Source: three-view drawing plus pictorial views. Frame: mm from the lowest corner of the part. A direction names the side the tool comes from. Give positions to 0.01 mm unless a question says otherwise; leave off trailing zeros. Loops run counter-clockwise (first coordinate to the right, second up) from the corner with the lowest first, then second, coordinate; pieces in that order, holes last.
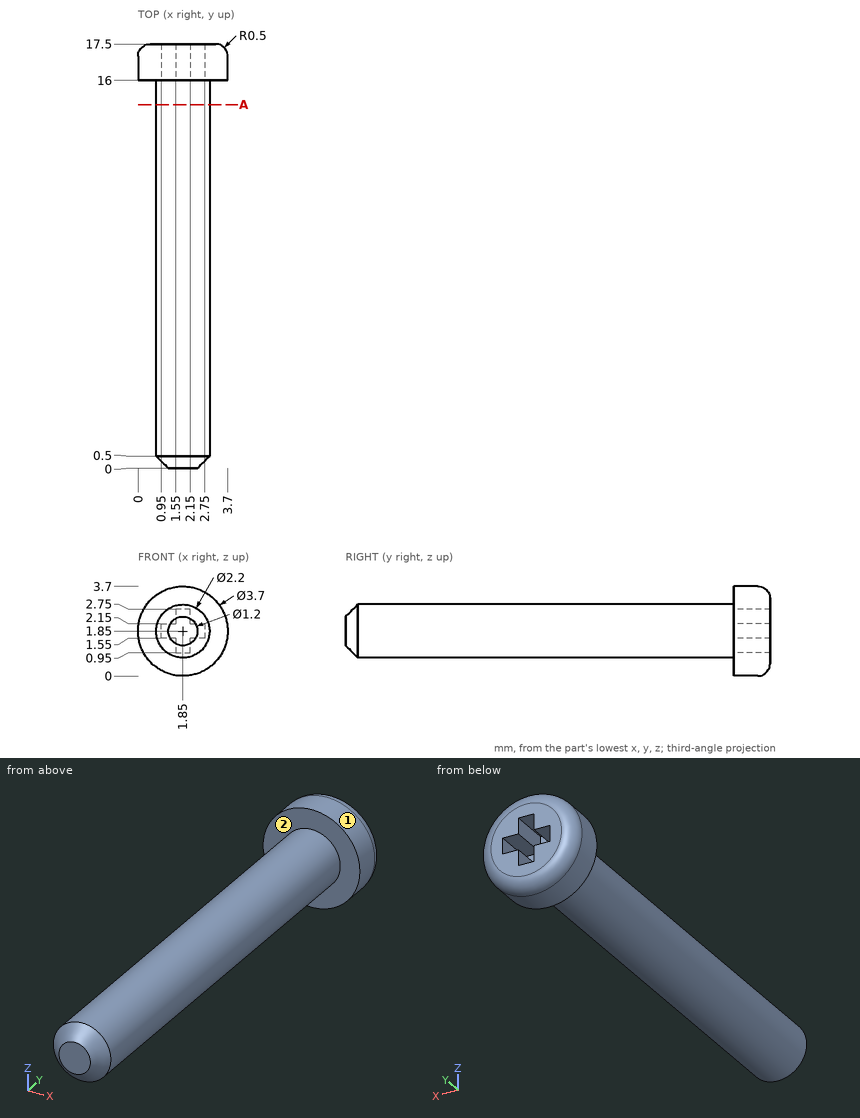
1) Ray query, probe 1 along X at (y, z) = (12.25, 1.8); probe 2 along Y at (x, z) = (3.2, 2.1); probe 3 along Y at (x, z) = (1.45, 1.75). Return the intervals inside material, ascending.
Checks:
probe 1: x = 0.75 to 2.95
probe 2: y = 16 to 17.5
probe 3: y = 0 to 16
2) Contact query for flat-ended pins moving along their axis: P1, Ø1.5, axis at y = 14, z = 1.5, coming from the +X side; P2, Ø1.5, axis at y = 4.5, z = 2, coming from the -X side; P3, Ø0.5, axis at x = 2.5, y = 17, coming from the +Z side. Output: stop coordinate, or through.
Checks:
P1: stops at x = 2.95
P2: stops at x = 0.75
P3: stops at z = 3.66
3) Reachability of the marked faces 1 and 2 from +Z, -Z, +X, -X, +Y, -Y: full face, straight path, thin tool, end or side. Return the list, or none.
Checks:
face 1: +Y, -Y
face 2: -Y
4) Cut plane A-A (y = 15). Return loops of the section in (x, z), and give its area (3 significant figures).
Checks:
outline: circle Ø2.2 at (1.85, 1.85)
area: 3.80 mm2
